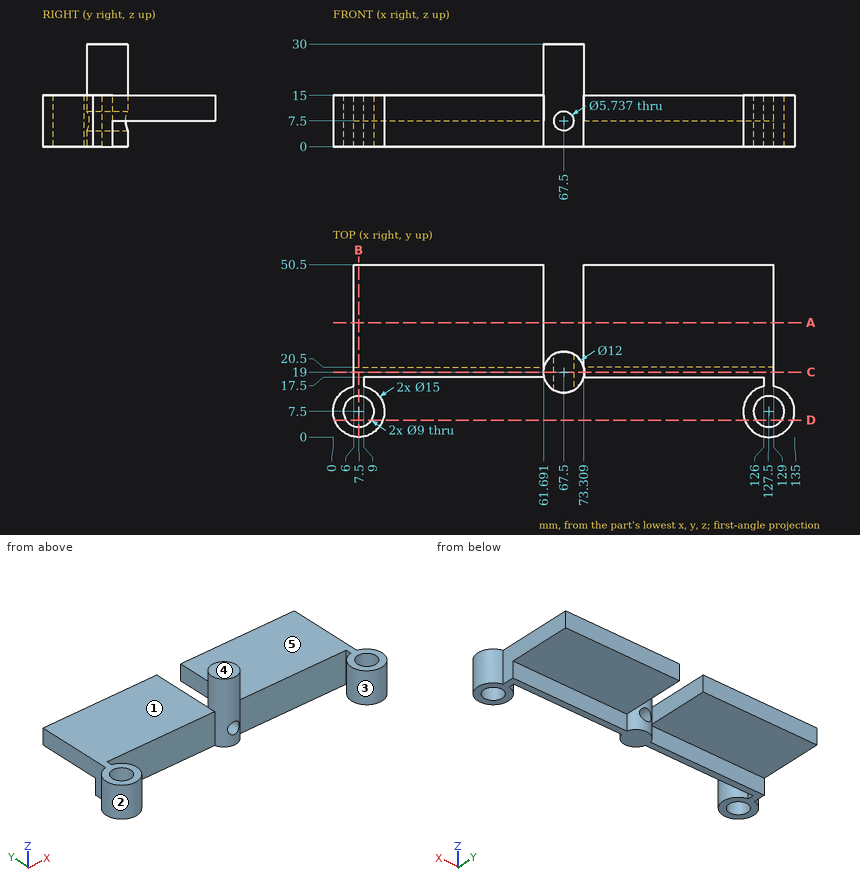
Print and shaded views of the part. All mm, measured from the part's lowest x, y and z. A direction names the side the tool comes from. Round coordinates to 2 decimals unless told otherwise and drop trailing zeros. Write each loop counter-clockwise with the first axis right and the second up, starting at its lowest first coordinate (ties: lowest second). Pieces come first, ordered by that corner, then holes.
(1) Mould opens along Y. For the marked faces 1, 2 and 3 say: pulls with the +Y half, pulls with the -Y half, needs draft (parallel to the pull), parting line crosses it, or undercut.
(2) Probe line 1 along X through (y, z) = (7, 7); line 2 along Y through (x, z) = (127.5, 6.5); line 3 along Y through (x, z) = (127, 11). List the from-to ranges inside material, lowest first.
(3) Slice it at C-C, the plane y = 19. Write the cut outline in (x, z).
(4) Drop flat-ended pins along their axis: P1, Ø4, axis at y = 9.5, z = 8.5, coming from the +X side; P2, Ø12, axis at x = 43.5, z = 10, coming from the -Y side; P3, Ø16.5, axis at y = 38.5, z = 8, coming from the -X side; P4, Ø4.5, axis at x = 67.5, z = 7.5, coming from the +Y side. Give the stop position or say it passes through.
(5) Slice it at A-A, the plane y = 33.5. Write the cut outline in (x, z).
(6) 3-axis set-ups, long thin cutter, end or side, ignore diameter. For the marked faces 4 and 5: which of +Z, -Z, +X, -X, +Y, -Y reach the whole face in a straight line?
(7) Slice it at B-B, the plane x = 7.5. Write the cut outline in (y, z).
(8) Slice it at D-D, the plane y = 5. Write the cut outline in (x, z), and give its area (3 significant figures).
From the geometry:
1. face 1: needs draft
1. face 2: undercut
1. face 3: undercut
2. line 1: x = 0.02 to 3.03, 11.97 to 14.98, 120.02 to 123.03, 131.97 to 134.98
2. line 2: y = 0 to 3, 12 to 20.5
2. line 3: y = 0.02 to 3.03, 11.97 to 50.5
3. outline: (6, 0) - (129, 0) - (129, 15) - (73.5, 15) - (73.5, 30) - (61.5, 30) - (61.5, 15) - (6, 15) - close; hole circle Ø5.74 at (67.5, 7.5)
4. P1: stops at x = 135
4. P2: stops at y = 17.5
4. P3: stops at x = 6
4. P4: passes through
5. outline: (6, 7.5) - (61.69, 7.5) - (61.69, 15) - (6, 15) - close; (73.31, 7.5) - (129, 7.5) - (129, 15) - (73.31, 15) - close
6. face 4: +Z, +X, -X, +Y, -Y
6. face 5: +Z, +X, +Y, -Y
7. outline: (0, 0) - (3, 0) - (3, 15) - (0, 15) - close; (12, 0) - (20.5, 0) - (20.5, 7.5) - (50.5, 7.5) - (50.5, 15) - (12, 15) - close
8. outline: (0.43, 0) - (3.76, 0) - (3.76, 15) - (0.43, 15) - close; (11.24, 0) - (14.57, 0) - (14.57, 15) - (11.24, 15) - close; (120.43, 0) - (123.76, 0) - (123.76, 15) - (120.43, 15) - close; (131.24, 0) - (134.57, 0) - (134.57, 15) - (131.24, 15) - close
8. area: 200 mm2
